```python
from build123d import *

# Parameters (mm, degrees)
FILLET1_R       = 0.1
SKETCH3_W       = 0.9
SKETCH3_H       = 3.5
SKETCH4_W       = 0.9
SKETCH4_H       = 1.754964664
RECPAT_COUNT    = 2
RECPAT_ANGLE    = 90
CHANFREIN1_SIZE = 0.3


with BuildPart() as part:
    # BodySke → Base-Revolve (revolve)
    with BuildSketch(Plane.XY):
        with BuildLine():
            Line((1.8, 1.5), (1.8, 2.55))
            Line((1.8, 2.55), (0.855787168, 2.55))
            ThreePointArc((0.855787168, 2.55), (0.718382578, 2.512421984), (0.619225336, 2.410147992))
            ThreePointArc((0.619225336, 2.410147992), (0.157280035, 1.244211935), (0, 0))
            Line((0, 0), (7.8, 0))
            Line((7.8, 0), (7.8, 1.5))
            Line((7.8, 1.5), (1.8, 1.5))
        make_face()
    revolve(axis=Axis((-25.4, 0, 0), (1, 0, 0)))

    # Fillet1
    fillet1_edges = [part.edges().sort_by_distance(p)[0] for p in [
        (1.8, -1.5, 0),
    ]]
    fillet(fillet1_edges, radius=FILLET1_R)

    # Sketch3 → Recess section 0
    with BuildSketch(Plane(origin=(0, 0, 0), x_dir=(0, 0, -1), z_dir=(1, 0, 0))):
        Rectangle(SKETCH3_W, SKETCH3_H)
    # Sketch4 → Recess section 1
    with BuildSketch(Plane(origin=(1.75, 0, 0), x_dir=(0, 0, -1), z_dir=(1, 0, 0))):
        Rectangle(SKETCH4_W, SKETCH4_H)
    recess = loft(mode=Mode.SUBTRACT)

    # RecPat: Recess ×2 about axis
    recpat_axis = Axis((0, 0, 0), (1, 0, 0))
    for i in range(1, RECPAT_COUNT):
        add(recess.rotate(recpat_axis, i * RECPAT_ANGLE / (RECPAT_COUNT - 1)), mode=Mode.SUBTRACT)

    # RecCorSke → RecessCore (revolve, cut)
    with BuildSketch(Plane.XY):
        Polygon((0, 0), (0, 0.678371921), (1.75, 0.556), (1.930655351, 0), align=None)
    revolve(axis=Axis((-3.175, 0, 0), (1, 0, 0)), mode=Mode.SUBTRACT)

    # Chanfrein1
    chanfrein1_edges = [part.edges().sort_by_distance(p)[0] for p in [
        (7.8, -1.5, 0),
    ]]
    chamfer(chanfrein1_edges, length=CHANFREIN1_SIZE)


solid = part.part
```
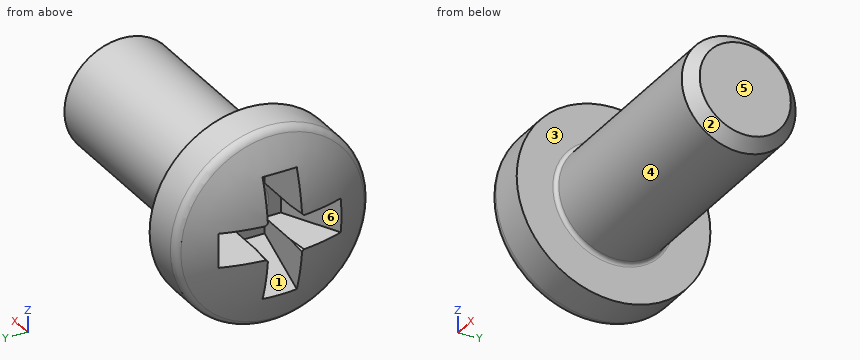
Can you work these out from the model? Positions are in its coordinate system, mm. Face numbers are marked on the shaded views. A direction names the side the tool comes from. Give positions to 0.01 mm unless a question says otherwise; leave off trailing zeros. Loops run counter-clockwise (first coordinate to the right, second up) from the corner with the lowest first, then second, coordinate; pieces in that order, holes last. Notation, with made-up numbers: M -4,11.5 L 17,11.5 A10 ccw 17,23.5 Z; hole C 26,37 d5. An arc over 180 degrees is marked long. One line per question, with ' | ' between items. Start each with the question number.
Q1. For pin 1 Ø1.5 at (x, y) = (7, 1) entering from -Z; pin 2 Ø2 at (x, z) = (6.5, -1.5) entering from -Y; pin 3 Ø1 at (x, y) = (6.5, -0.5) entering from +Z; pin 4 Ø2 at (x, z) = (2, -1) entering from -Y, each with a flat end and sliding along its axis, tell me the tip position at first contact or that it passes through.
Q2. If I drill on line 1 (Z direction, x = 1.5, y = -0.2); line 2 (Y direction, x = 1.25, z = -0.35); line 3 (Y direction, x = 5, z = 0.05), over which ranges is the centre line in solid material (lowest first)? Write a range as from..to.
Q3. For the marked faces 4, 5 and 6, which set-ups out of +Z, -Z, +X, -X, +Y, -Y let a thin tool reach every point of the face, with its end or its side?
Q4. If we mould it in two halves opening along Z, with no side actions, what happens to the marked faces 1, 2 and 3? For each: +Z half, -Z half, draft (parallel to the pull), parting line (faces both ways), or undercut.
Q5. If we section it at A-A (x = 5): Please give me the cut outline in (y, z), plus the area to 3 significant figures.
Computed:
1) pin 1: stops at z = -1.48 | pin 2: stops at y = -1.41 | pin 3: stops at z = 1.5 | pin 4: stops at y = -2.55
2) line 1: z = -2.54..-1, 1..2.54 | line 2: y = -2.53..-1.13, 1.13..2.53 | line 3: y = -1.5..1.5
3) face 4: +X | face 5: +Z, -Z, +X, +Y, -Y | face 6: -X
4) face 1: undercut | face 2: parting line | face 3: draft
5) outline: C 0,0 d3 | area: 7.07 mm²
